```python
from build123d import *

# Parameters (mm, degrees)
F0_W     = 370
F0_H     = 320
F1_DEPTH = 70
F2_W     = 322.659016
F2_H     = 252.088964
F3_DEPTH = 60
F4_W     = 342
F4_H     = 140
F5_DEPTH = 26


with BuildPart() as f1:
    # F0 (on Top) → F1 (new body)
    with BuildSketch(Plane.XY):
        Rectangle(F0_W, F0_H)
    extrude(amount=F1_DEPTH)

    # F2 (on face) → F3 (cut)
    with BuildSketch(Plane.XY.offset(70)):
        Rectangle(F2_W, F2_H)
    extrude(amount=-F3_DEPTH, mode=Mode.SUBTRACT)

    # F4 (on face) → F5 (join)
    with BuildSketch(Plane.YZ.offset(185)):
        with Locations((0, 25.815584)):
            Rectangle(F4_W, F4_H)
    extrude(amount=F5_DEPTH)


solid = f1.part
```
The listing builds one solid part. Answer for the finished solid, in the listing's coordinates (mm). A direction names the side the tool comes from. Round coordinates to 2 decimals unless told otherwise and drop trailing zeros. Loops run counter-clockwise (first coordinate to the right, second up) from the corner with the lowest first, then second, coordinate; pieces in that order, holes last.
1) A cutting plane is placed at C-C on z = 61.5. Determine the outline of the cut face in (x, y).
Outcome:
outline: (-185, -160) - (185, -160) - (185, -171) - (211, -171) - (211, 171) - (185, 171) - (185, 160) - (-185, 160) - close; hole (-161.33, -126.04) - (161.33, -126.04) - (161.33, 126.04) - (-161.33, 126.04) - close
2) A cutting plane is placed at B-B on x = -70.5. Determine the outline of the cut face in (y, z).
Outcome:
outline: (-160, 0) - (160, 0) - (160, 70) - (126.04, 70) - (126.04, 10) - (-126.04, 10) - (-126.04, 70) - (-160, 70) - close
3) Given P1, Ø3, axis at x = 68, y = 39.5, coming from the +Z side; P2, Ø1.5, axis at x = 84.5, z = 57, coming from the +Y side; P3, Ø12, axis at y = -12.5, z = -12, coming from the -X side, each flat-ended and moving along its own axis, determine where each tip first touches the part or whether it passes through.
Outcome:
P1: stops at z = 10
P2: stops at y = 160
P3: stops at x = 185
4) A cutting plane is placed at A-A on y = 61.5. Determine the outline of the cut face in (x, z).
Outcome:
outline: (-185, 0) - (185, 0) - (185, -44.18) - (211, -44.18) - (211, 95.82) - (185, 95.82) - (185, 70) - (161.33, 70) - (161.33, 10) - (-161.33, 10) - (-161.33, 70) - (-185, 70) - close
5) For a pull along Y with two mould halves and no side action, classify faces 4 (the face through (-2, 126.044, 40)), 5 (the face through (198, 171, 25)), 6 (the face through (-2, -126.044, 40)), 7 (the face through (198, -2, 95.816)) as released by +Y, released by -Y, zero draft, split by the parting line, or undercut.
Outcome:
face 4: undercut
face 5: released by +Y
face 6: undercut
face 7: zero draft
6) Consider line 1 (Y direction, x = 15, z = 67.5); line 2 (Z direction, x = 69.5, y = 128); line 3 (Z direction, x = 159.5, y = -70). Determine where each line is inside the solid, lowest interval first.
Outcome:
line 1: y = -160 to -126.04, 126.04 to 160
line 2: z = 0 to 70
line 3: z = 0 to 10
7) For faces 1 (the face through (-3, 160, 35)), 2 (the face through (-161.33, -2, 40)), 3 (the face through (-3, -160, 35)), determine the directions among +Z, -Z, +X, -X, +Y, -Y from which every point of the face is accessible in a straight line to the end or side of a thin tool.
Outcome:
face 1: +Z, -Z, -X, +Y
face 2: +Z
face 3: +Z, -Z, -X, -Y
